Autodesk Inventor part; units mm, degrees
ref_plane "YZ Plane" through (0, 0, 0) normal (1, 0, 0) x (0, 1, 0)
ref_plane "XZ Plane" through (0, 0, 0) normal (0, 1, 0) x (-1, 0, 0)
ref_plane "XY Plane" through (0, 0, 0) normal (0, 0, 1) x (1, 0, 0)
sketch "Sketch1" plane through (0, 0, 0) normal (0, 1, 0) x (-1, 0, 0)
  line L0 (7, 8.75) -> (-7, 8.75)
  line L1 (-7, 8.75) -> (-7, -8.75)
  line L2 (-7, -8.75) -> (7, -8.75)
  line L3 (7, -8.75) -> (7, 8.75)
  point P0 (0, 0)
  point P1 (0, -8.75)
  point P2 (-7, 0)
  dimension "d0" = 17.5
  dimension "d1" = 14
extrude "Extrusion1" add sketch "Sketch1" along normal blind 1.6
sketch "Sketch2" plane through (0, 1.6, 0) normal (0, 1, 0) x (1, 0, 0)
  line L0 (0, 3.5818) -> (0, 1.7058) construction
  line L1 (-7, -8.75) -> (7, -8.75) construction
  point P0 (0, 0)
  point P1 (0, -1.25)
  point P2 (-3.81, 6.75)
  point P3 (-1.27, 6.75)
  point P4 (1.27, 6.75)
  point P5 (3.81, 6.75)
  point P6 (-2.54, -6.75)
  point P7 (0, -6.75)
  point P8 (2.54, -6.75)
  dimension "d4" = 2.54
  dimension "d5" = 2.54
  dimension "d7" = 2.54
  dimension "d8" = 5.5
  dimension "d9" = 8
  dimension "d10" = 2
hole "Hole1" at (-3.81, 1.6, -6.75) at (-1.27, 1.6, -6.75) at (1.27, 1.6, -6.75) at (3.81, 1.6, -6.75) at (-2.54, 1.6, 6.75) at (0, 1.6, 6.75) at (2.54, 1.6, 6.75) direction (0, -1, 0) diameter 0.5 end through all
sketch "Sketch3" plane through (0, 1.6, 0) normal (0, 1, 0) x (1, 0, 0)
  circle A0 centre (0, -1.25) radius 2.5
  circle A1 centre (0, -6.75) radius 0.25
  point P0 (0, 0)
  dimension "d20" = 5.5
  dimension "d21" = 5
sketch "Sketch4" plane through (0, 1.6, 0) normal (0, 1, 0) x (1, 0, 0)
  point P0 (0, 0)
extrude "Extrusion2" add sketch "Sketch3" along normal blind 8.5 contours A0
fillet "Fillet1" radius 2.5 1 edges at (-2.5, 10.1, 1.25)
sketch "Sketch5" plane through (0, 1.6, 0) normal (0, 1, 0) x (1, 0, 0)
  circle A0 centre (0, -1.25) radius 2.5
  arc A1 (-2.5, -3.3267) -> (-2.5, 0.8267) centre (0, -1.25) ccw
  line L0 (-2.5, 0.8267) -> (-2.5, -3.3267)
  point P0 (0, 0)
  point P1 (-2.5, -1.25)
  dimension "d23" = 6.5
extrude "Extrusion3" add sketch "Sketch5" along normal blind 1
properties part number "LED_module"
The model under review builds one solid part; all positions refer to its coordinate system, in mm. A direction names the side the tool comes from. Give positions to 0.01 mm unless a question says otherwise; leave off trailing zeros. Write each loop counter-clockwise with the first axis right and the second up, starting at its lowest first coordinate (ties: lowest second). Pieces come first, ordered by that corner, then holes. Notation, with made-up numbers: (9.5, -22) -> (26.5, -22) arc R30 ccw to (26.5, 3) -> close; hole circle Ø2 at (24, 56). An arc over 180 degrees is marked (long way). Put each result on its own line as item: value.
(1) To check wall thickness, follow probe 1 along X at (y, z) = (0.55, -6.75); probe 2 along X at (y, z) = (1.05, 6.75); probe 3 along Z at (x, y) = (-3.81, 0.65). State the ranges of each line that lie inside material, in increasing order. Write a range as from..to.
Results are:
probe 1: -7..-4.06, -3.56..-1.52, -1.02..1.02, 1.52..3.56, 4.06..7
probe 2: -7..-2.79, -2.29..-0.25, 0.25..2.29, 2.79..7
probe 3: -8.75..-7, -6.5..8.75
(2) We need section A-A, the plane x = -3.81. Give the boundary of the cut face in (y, z), and give its area (3 significant figures).
Results are:
outline: (0, -8.75) -> (1.6, -8.75) -> (1.6, -7) -> (0, -7) -> close; (0, -6.5) -> (1.6, -6.5) -> (1.6, 8.75) -> (0, 8.75) -> close
area: 27.2 mm²
(3) Tool access review of faces 1 (the flat face through (-2.5, 2, 1)), 2 (the flat face through (0, 1, 8.75)), 3 (the flat face through (2, 1.6, -2)): name each direction out of +Z, -Z, +X, -X, +Y, -Y from which nothing blocks a thin tool from reaching the whole face with its end or side.
Results are:
face 1: +Z, -Z, -X, +Y
face 2: +Z, +X, -X, +Y, -Y
face 3: +Y
(4) For pin 1 Ø3 at (y, z) = (9, 1) entering from +X; pin 2 Ø3 at (x, z) = (-5, 3.5) entering from +Y; pin 3 Ø1 at (x, z) = (-2.5, 2.5) entering from +Y, all flat-tipped, find the tip position at first contact; note any pin that passes through.
Results are:
pin 1: x = 2.5
pin 2: y = 1.6
pin 3: y = 8.59
(5) We need section C-C, the plane x = -1.27. Give the boundary of the cut face in (y, z), and give its area (3 significant figures).
Results are:
outline: (0, -8.75) -> (1.6, -8.75) -> (1.6, -7) -> (0, -7) -> close; (0, -6.5) -> (1.6, -6.5) -> (1.6, -1.74) -> (2.6, -1.74) -> (2.6, -0.9) -> (7.6, -0.9) arc R2.15 ccw to (7.6, 3.4) -> (2.6, 3.4) -> (2.6, 4.24) -> (1.6, 4.24) -> (1.6, 8.75) -> (0, 8.75) -> close
area: 62.0 mm²
(6) We need section D-D, the plane z = 2.75. Give the boundary of the cut face in (x, y).
Results are:
outline: (-7, 0) -> (7, 0) -> (7, 1.6) -> (2.88, 1.6) -> (2.88, 2.6) -> (2, 2.6) -> (2, 7.6) arc R2 ccw to (-2, 7.6) -> (-2, 2.6) -> (-2.5, 2.6) -> (-2.5, 1.6) -> (-7, 1.6) -> close
(7) We need section B-B, the plane z = 6.75. Give the boundary of the cut face in (x, y).
Results are:
outline: (-7, 0) -> (-2.79, 0) -> (-2.79, 1.6) -> (-7, 1.6) -> close; (-2.29, 0) -> (-0.25, 0) -> (-0.25, 1.6) -> (-2.29, 1.6) -> close; (0.25, 0) -> (2.29, 0) -> (2.29, 1.6) -> (0.25, 1.6) -> close; (2.79, 0) -> (7, 0) -> (7, 1.6) -> (2.79, 1.6) -> close
